```python
from build123d import *

# Parameters (mm, degrees)
PROFILEBOSS_EXTRUDE1_DEPTH         = 15
SKETCH2_R                          = 2.5
MOUNTHOLESCUT_EXTRUDE1_DEPTH       = 52.877258987
CHAMFER1_SIZE                      = 1.1
GROMMETHOLECUT_EXTRUDE2_REACH      = 49.053
GROMMETHOLECUT_EXTRUDE2_END_RADIUS = 4
SKETCH3_R                          = 2.5


with BuildPart() as part:
    # Sketch1 → ProfileBoss-Extrude1 (new body)
    with BuildSketch(Plane(origin=(0, 0, 0), x_dir=(0, 0, -1), z_dir=(1, 0, 0))):
        with BuildLine():
            Line((0, 0), (42, 0))
            Line((42, 0), (42, 6.5))
            Line((42, 6.5), (30, 6.5))
            Line((30, 6.5), (30, 33))
            Line((30, 33), (21.5, 33))
            Line((21.5, 33), (21.5, 23.718626967))
            ThreePointArc((21.5, 23.718626967), (21, 15.75), (20.5, 23.718626967))
            Line((20.5, 23.718626967), (20.5, 33))
            Line((20.5, 33), (12, 33))
            Line((12, 33), (12, 6.5))
            Line((12, 6.5), (0, 6.5))
            Line((0, 6.5), (0, 0))
        make_face()
    extrude(amount=PROFILEBOSS_EXTRUDE1_DEPTH)

    # Sketch2 → MountHolesCut-Extrude1 (cut, through all)
    with BuildSketch(Plane(origin=(0, 6.5, 0), x_dir=(1, 0, 0), z_dir=(0, 1, 0))):
        with Locations(Location((7.5, 5.5, 0), (0, 0, 270))):
            Circle(SKETCH2_R)
        with Locations(Location((7.5, 36.5, 0), (0, 0, 270))):
            Circle(SKETCH2_R)
    extrude(amount=-MOUNTHOLESCUT_EXTRUDE1_DEPTH, mode=Mode.SUBTRACT)

    # Chamfer1
    chamfer1_edges = [part.edges().sort_by_distance(p)[0] for p in [
        (7.5, 6.5, -8),
        (7.5, 6.5, -39),
    ]]
    chamfer(chamfer1_edges, length=CHAMFER1_SIZE)

    # GrommetHoleCut-Extrude2: up to this cylinder (the profile starts outside it)
    grommetholecut_extrude2_end = Plane(origin=(7.5, 19.75, -21), z_dir=(-1, 0, 0)) * Cylinder(GROMMETHOLECUT_EXTRUDE2_END_RADIUS, 107.106, mode=Mode.PRIVATE)
    # Sketch3 → GrommetHoleCut-Extrude2 (cut, up to the surface)
    with BuildSketch(Plane.XY.offset(-12), mode=Mode.PRIVATE) as grommetholecut_extrude2_sk1:
        with Locations((7.5, 19.75)):
            Circle(SKETCH3_R)
    grommetholecut_extrude2_tool1 = extrude(grommetholecut_extrude2_sk1.sketch, amount=-GROMMETHOLECUT_EXTRUDE2_REACH, mode=Mode.PRIVATE) - grommetholecut_extrude2_end
    add(grommetholecut_extrude2_tool1.solids().sort_by_distance((7.5, 19.75, -12))[0], mode=Mode.SUBTRACT)


solid = part.part
```
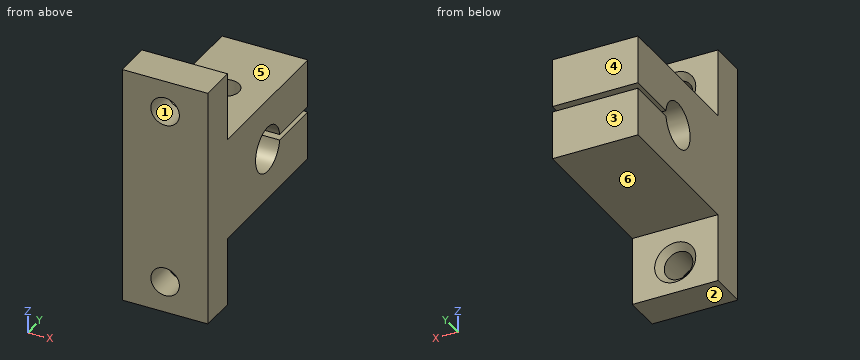
Check sheet for the modelled part. Datum: model origin and axes. Units: mm. Face numbers are marked on the shaded views. A direction names the side the tool comes from. Round coordinates to 2 decimals unless told otherwise and drop trailing zeros. Loops run counter-clockwise (first coordinate to the right, second up) from the corner with the lowest first, then second, coordinate; pieces in that order, holes last. Notation, with made-up numbers: (24, -36.75) -> (45, -36.75) arc R9 ccw to (45, -19.75) -> close; hole circle Ø1 at (-16.5, -30). An arc over 180 degrees is marked (long way). Write item = value, one per line. Start each with the question number.
1) Sectioned sample at C-C, the plane x = 7.5. Record the cut outline in (y, z), plus the area to 3 significant figures.
2) Release check for a two-part mould opening along Z. For the marked faces 1, 2 and 3 record: released by +Z, released by -Z, zero draft, split by the parting line, or undercut.
3) Sectioned sample at B-B, the plane y = 30.5. Record the cut outline in (x, z), plus the area to 3 significant figures.
4) Gauge pin test, flat ends, axial feed: pin 1 Ø4 at (x, z) = (8, -7) entering from -Y; pin 2 Ø5 at (x, z) = (3, -33) entering from +Y; pin 3 Ø3 at (x, y) = (11, 29.5) entering from +Z; pin 4 Ø4.5 at (x, y) = (7.5, 19.75) entering from +Z. Record the tip position at first contact, or that the pin passes through.
5) Sectioned sample at A-A, the plane z = -36.5. Record the cut outline in (x, y), plus the area to 3 significant figures.
6) Set-up check for the marked faces 4, 5 and 6: record each of +Z, -Z, +X, -X, +Y, -Y from which the full face is reachable in a straight line by a thin tool's end or side.
7) Thickness scan on probe 1 along Y at (x, z) = (7.5, -13.5); probe 2 along X at (y, z) = (1.1, -36.5); probe 3 along Z at (x, y) = (11.75, 24). Record the ranges inside material, lowest first.
8) Sectioned sample at D-D, the plane y = 4. Record the cut outline in (x, z).
Results are:
q1.outline = (0, -42) -> (6.5, -42) -> (6.5, -40.1) -> (5.4, -39) -> (0, -39) -> close; (0, -34) -> (5.4, -34) -> (6.5, -32.9) -> (6.5, -30) -> (33, -30) -> (33, -21.5) -> (23.72, -21.5) arc R4 cw (long way) to (17.25, -17.88) -> (17.25, -12) -> (6.5, -12) -> (6.5, -9.1) -> (5.4, -8) -> (0, -8) -> close; (0, -3) -> (5.4, -3) -> (6.5, -1.9) -> (6.5, 0) -> (0, 0) -> close; (22.25, -17.88) arc R4 cw to (23.72, -20.5) -> (33, -20.5) -> (33, -12) -> (22.25, -12) -> close
q1.area = 597 mm^2
q2.face_1 = undercut
q2.face_2 = released by -Z
q2.face_3 = zero draft
q3.outline = (0, -30) -> (15, -30) -> (15, -21.5) -> (0, -21.5) -> close; (0, -20.5) -> (15, -20.5) -> (15, -12) -> (0, -12) -> close
q3.area = 255 mm^2
q4.pin_1 = 0
q4.pin_2 = 6.5
q4.pin_3 = -12
q4.pin_4 = -24.31
q5.outline = (0, 0) -> (5, 0) -> (5, 5.4) -> (3.9, 6.5) -> (0, 6.5) -> close; (10, 0) -> (15, 0) -> (15, 6.5) -> (11.1, 6.5) -> (10, 5.4) -> close
q5.area = 63.8 mm^2
q6.face_4 = +Z, -Z, +X, -X, +Y
q6.face_5 = +Z, +X, -X, +Y
q6.face_6 = -Z, +X, -X, +Y
q7.probe_1 = 0 to 17.25, 22.25 to 33
q7.probe_2 = 0 to 5, 10 to 15
q7.probe_3 = -30 to -21.5, -20.5 to -12
q8.outline = (0, -42) -> (15, -42) -> (15, 0) -> (0, 0) -> close; hole circle Ø5 at (7.5, -36.5); hole circle Ø5 at (7.5, -5.5)
